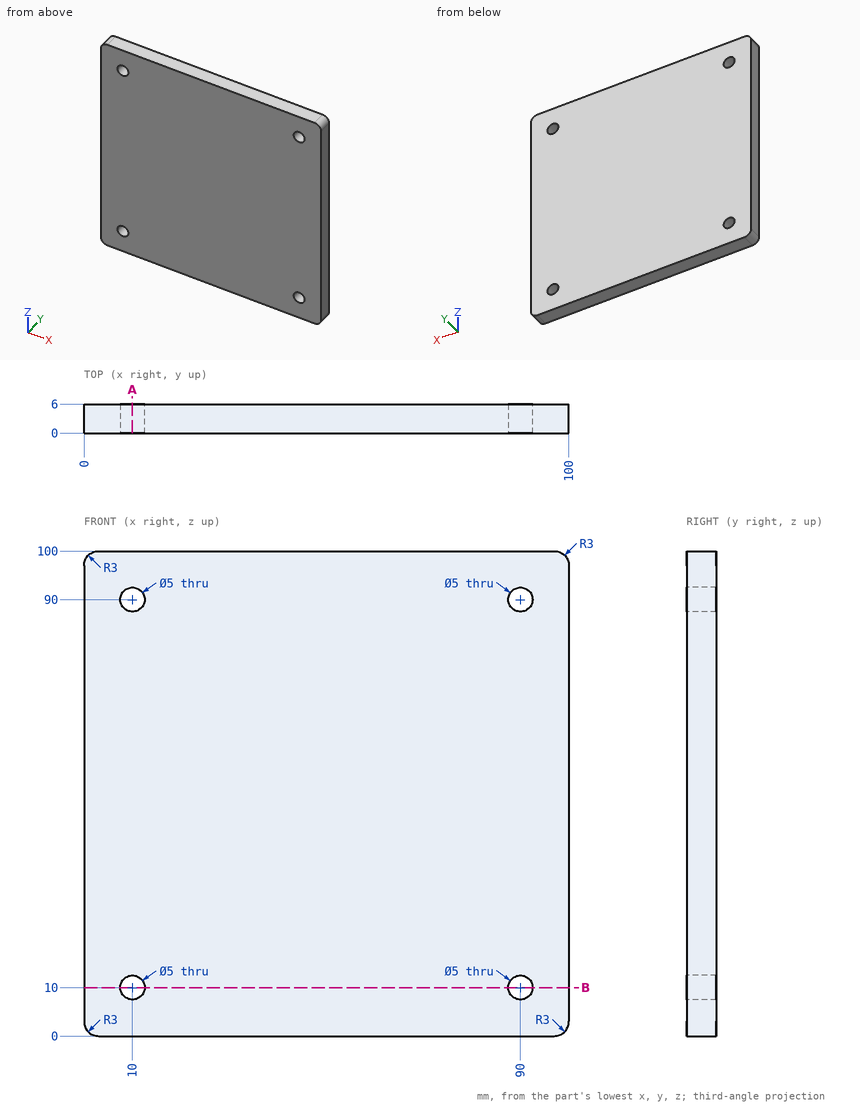
Geometry check sheet. Reference: drawing and pictorial views, mm from the part's lowest x, y, z. Coordinates: 2 decimals unless noted, no trailing zeros. Order: outer loops, then holes, each group sorted by start corner. A loop starts at its lowest first (then second) coordinate and runs counter-clockwise, first axis right, second up.
Item 1: Section check A-A (x = 10). Enter the section's corners in (y, z).
Item 2: Scan lines: line 1 along Z through (x, y) = (10, 2.35); line 2 along Z through (x, y) = (8, 1.7). Record each from-to range of solid material in increasing order.
Item 3: Section check B-B (z = 10). Enter the section's corners in (x, y).
Check sheet entries:
1. outline: (0, 0) - (6, 0) - (6, 7.5) - (0, 7.5) - close; (0, 12.5) - (6, 12.5) - (6, 87.5) - (0, 87.5) - close; (0, 92.5) - (6, 92.5) - (6, 100) - (0, 100) - close
2. line 1: z = 0 to 7.5, 12.5 to 87.5, 92.5 to 100
2. line 2: z = 0 to 8.5, 11.5 to 88.5, 91.5 to 100
3. outline: (0, 0) - (7.5, 0) - (7.5, 6) - (0, 6) - close; (12.5, 0) - (87.5, 0) - (87.5, 6) - (12.5, 6) - close; (92.5, 0) - (100, 0) - (100, 6) - (92.5, 6) - close
